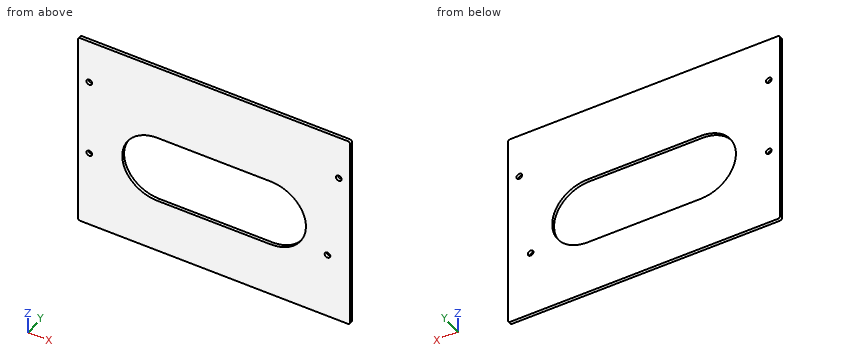
```python
from build123d import *

# Parameters (mm, degrees)
BOSS_EXTRUDE1_DEPTH = 3.5
CUT_EXTRUDE7_DEPTH  = 289.878374321
SKETCH8_R           = 3.175
CUT_EXTRUDE8_DEPTH  = 289.878374321


with BuildPart() as part:
    # Sketch1 → Boss-Extrude1 (new body)
    with BuildSketch(Plane(origin=(0, 0, 0), x_dir=(1, 0, 0), z_dir=(0, 1, 0))):
        with BuildLine():
            Line((-126.953423408, -0.978024545), (172.766576592, -0.978024545))
            ThreePointArc((172.766576592, -0.978024545), (174.562627816, -1.721973321), (175.306576592, -3.518024545))
            Line((175.306576592, -3.518024545), (175.306576592, -227.038024545))
            ThreePointArc((175.306576592, -227.038024545), (174.562627816, -228.834075769), (172.766576592, -229.578024545))
            Line((172.766576592, -229.578024545), (-126.953423408, -229.578024545))
            ThreePointArc((-126.953423408, -229.578024545), (-128.749474632, -228.834075769), (-129.493423408, -227.038024545))
            Line((-129.493423408, -227.038024545), (-129.493423408, -3.518024545))
            ThreePointArc((-129.493423408, -3.518024545), (-128.749474632, -1.721973321), (-126.953423408, -0.978024545))
        make_face()
    extrude(amount=BOSS_EXTRUDE1_DEPTH)

    # Sketch7 → Cut-Extrude7 (cut, through all)
    with BuildSketch(Plane(origin=(0, 0, 0), x_dir=(-1, 0, 0), z_dir=(0, -1, 0))):
        with BuildLine():
            Line((40.593423408, -141.948024545), (-86.406576592, -141.948024545))
            ThreePointArc((-86.406576592, -141.948024545), (-125.776576592, -102.578024545), (-86.406576592, -63.208024545))
            Line((-86.406576592, -63.208024545), (40.593423408, -63.208024545))
            ThreePointArc((40.593423408, -63.208024545), (79.963423408, -102.578024545), (40.593423408, -141.948024545))
        make_face()
    extrude(amount=-CUT_EXTRUDE7_DEPTH, mode=Mode.SUBTRACT)

    # Sketch8 → Cut-Extrude8 (cut, through all)
    with BuildSketch(Plane(origin=(0, 0, 0), x_dir=(-1, 0, 0), z_dir=(0, -1, 0))):
        with Locations(Location((-149.906576592, -77.178024545, 0), (0, 0, 90))):
            Circle(SKETCH8_R)
        with Locations(Location((116.793423408, -89.878024545, 0), (0, 0, 90))):
            Circle(SKETCH8_R)
        with Locations(Location((116.793423408, -178.778024545, 0), (0, 0, 90))):
            Circle(SKETCH8_R)
        with Locations(Location((-162.606576592, -178.778024545, 0), (0, 0, 90))):
            Circle(SKETCH8_R)
    extrude(amount=-CUT_EXTRUDE8_DEPTH, mode=Mode.SUBTRACT)


solid = part.part
```
Work out the finished part from the listing and answer in its coordinate system (mm). Round coordinates to 2 decimals unless told otherwise and drop trailing zeros. Write each loop counter-clockwise with the first axis right and the second up, starting at its lowest first coordinate (ties: lowest second). Pieces come first, ordered by that corner, then holes. Notation, with made-up numbers: (1, 43) - (11, 43) arc R23 ccw to (11, 76) - close; hole circle Ø11 at (52.25, 23.5). An arc over 180 degrees is marked (long way). Return JSON: item names as keys, results as strings. Group by question number.
Q1. This flat-tipped pin is pushed along its axis until it touches: pin 1 Ø5.5 at (x, z) = (-116.79, 178.78) entering from +Y. Where does it stop, or does it pass through?
Q2. The part is cut by section A-A on x = 24. Write down the section's boundary in (y, z).
Q3. Find the intervals of material crossed by L1, parallel to Z at x = 7.5, y = 2.4; L2, parallel to X at y = 1.65, z = 88; L3, parallel to X at y = 2.55, z = 79, in increasing order.
Q4. The part is cut by section B-B on z = 130. Write down the section's boundary in (x, y).
Q5. The part is cut by section C-C on y = 1.65. Write down the section's boundary in (x, z) (3 decimals).
Solved:
{
 "1": {"pin 1": "through"},
 "2": {"outline": "(0, 0.98) - (3.5, 0.98) - (3.5, 63.21) - (0, 63.21) - close; (0, 141.95) - (3.5, 141.95) - (3.5, 229.58) - (0, 229.58) - close"},
 "3": {"L1": "0.98 to 63.21, 141.95 to 229.58", "L2": "-129.49 to -119.35, -114.23 to -77.16, 122.98 to 175.31", "L3": "-129.49 to -72.12, 117.94 to 147.31, 152.51 to 175.31"},
 "4": {"outline": "(-129.49, 0) - (-68.84, 0) - (-68.84, 3.5) - (-129.49, 3.5) - close; (114.66, 0) - (175.31, 0) - (175.31, 3.5) - (114.66, 3.5) - close"},
 "5": {"outline": "(-129.493, 3.518) arc R2.54 ccw to (-126.953, 0.978) - (172.767, 0.978) arc R2.54 ccw to (175.307, 3.518) - (175.307, 227.038) arc R2.54 ccw to (172.767, 229.578) - (-126.953, 229.578) arc R2.54 ccw to (-129.493, 227.038) - close; hole circle Ø6.35 at (-116.793, 89.878); hole circle Ø6.35 at (-116.793, 178.778); hole (-40.593, 63.208) - (86.407, 63.208) arc R39.37 ccw to (86.407, 141.948) - (-40.593, 141.948) arc R39.37 ccw to start; hole circle Ø6.35 at (149.907, 77.178); hole circle Ø6.35 at (162.607, 178.778)"}
}
